Autodesk Inventor part; units mm, degrees
ref_plane "YZ Plane" through (0, 0, 0) normal (1, 0, 0) x (0, 1, 0)
ref_plane "XZ Plane" through (0, 0, 0) normal (0, 1, 0) x (-1, 0, 0)
ref_plane "XY Plane" through (0, 0, 0) normal (0, 0, 1) x (1, 0, 0)
sketch "Sketch5" plane through (0, 0, 0) normal (0, 1, 0) x (-1, 0, 0)
  line L0 (0, 0) -> (40, 0)
  line L1 (40, 0) -> (40, 150)
  line L2 (40, 150) -> (0, 150)
  line L3 (0, 150) -> (0, 0)
  line L4 (40, 150) -> (40, 140)
  line L5 (40, 140) -> (30, 140)
  circle A0 centre (30, 140) radius 2.75
  circle A1 centre (30, 10) radius 2.75
  circle A2 centre (10, 140) radius 2.75
  circle A3 centre (10, 10) radius 2.75
  line L6 (32.75, 140) -> (32.75, 10)
  line L7 (27.25, 10) -> (27.25, 140)
  line L8 (12.75, 140) -> (12.75, 10)
  line L9 (7.25, 10) -> (7.25, 140)
  dimension "d107" = 40
  dimension "d108" = 150
  dimension "d109" = 10
  dimension "d110" = 10
  dimension "d111" = 5.5
  dimension "d114" = 130
  dimension "d117" = 20
extrude "Extrusion3" add sketch "Sketch5" along normal blind 10
sketch "Sketch6" plane through (0, 10, 0) normal (0, 1, 0) x (1, 0, 0)
  arc A0 (-32.75, -140) -> (-27.25, -140) centre (-30, -140) ccw
  circle A1 centre (-30, -140) radius 4.5
  arc A2 (-27.25, -10) -> (-32.75, -10) centre (-30, -10) ccw
  circle A3 centre (-30, -10) radius 4.5
  arc A4 (-7.25, -10) -> (-12.75, -10) centre (-10, -10) ccw
  circle A5 centre (-10, -10) radius 4.5
  circle A6 centre (-10, -140) radius 4.5
  line L0 (-34.5, -140) -> (-34.5, -10)
  line L1 (-25.5, -10) -> (-25.5, -140)
  line L2 (-14.5, -140) -> (-14.5, -10)
  line L3 (-5.5, -10) -> (-5.5, -140)
  point P0 (0, 0)
  dimension "d122" = 9
  dimension "d123" = 9
  dimension "d124" = 9
  dimension "d125" = 9
extrude "Extrusion4" cut sketch "Sketch6" against normal blind 6
fillet "Fillet2" radius 5 4 edges at (0, 5, 150) (-40, 5, 150) (0, 5, 0) (-40, 5, 0)
properties part number "GARFO" material "Aluminium AW-7020"
Can you work these out from the model? Positions are in its coordinate system, mm. A direction names the side the tool comes from. Coordinates: 2 decimals unless noted, no trailing zeros. Write each loop counter-clockwise with the first axis right and the second up, starting at its lowest first coordinate (ties: lowest second). Pieces come first, ordered by that corner, then holes. Notation, with made-up numbers: (75.5, 37) - (81.5, 37) arc R11 ccw to (81.5, 44) - close; hole circle Ø10 at (24.5, -19). An arc over 180 degrees is marked (long way). Return JSON: item names as keys, results as strings.
Q1. If we section it at B-B (y = 5.25): Please give me the cut outline in (x, z), then the cut area to 3 significant figures.
Computed values:
{"outline": "(-40, 5) arc R5 ccw to (-35, 0) - (-5, 0) arc R5 ccw to (0, 5) - (0, 145) arc R5 ccw to (-5, 150) - (-35, 150) arc R5 ccw to (-40, 145) - close; hole (-34.5, 10) arc R4.5 ccw to (-25.5, 10) - (-25.5, 140) arc R4.5 ccw to (-34.5, 140) - close; hole (-14.5, 10) arc R4.5 ccw to (-5.5, 10) - (-5.5, 140) arc R4.5 ccw to (-14.5, 140) - close", "area": "3,510 mm2"}
Q2. Thinking about a two-plate mould opening in Z: for faces 1 (the cylindrical face through (-2, 5, 149)), 2 (the cylindrical face through (-1, 5, 2)), 3 (the flat face through (-33, 4, 74)), which applies, +Z half, -Z half, draft (parallel to the pull), parting line (faces both ways), or undercut?
Computed values:
{"face 1": "+Z half", "face 2": "-Z half", "face 3": "undercut"}
Q3. On a 3-axis mill with a long thin cutter (end or side, diameter ignored), from which of +Z, -Z, +X, -X, +Y, -Y can I reach the whole of each face in a straight line? I mean faces 4 (the flat face through (-20, 5, 150)), 5 (the cylindrical face through (-29.9, 7, 5.5)), 6 (the cylindrical face through (-9.94, 1.97, 142.75)). Say none if no direction works.
Computed values:
{"face 4": "+Z, +X, -X, +Y, -Y", "face 5": "+Y", "face 6": "+Y, -Y"}
Q4. If we section it at A-A (z = 104): Please give me the cut outline in (x, y).
Computed values:
{"outline": "(-40, 0) - (-32.75, 0) - (-32.75, 4) - (-34.5, 4) - (-34.5, 10) - (-40, 10) - close; (-27.25, 0) - (-12.75, 0) - (-12.75, 4) - (-14.5, 4) - (-14.5, 10) - (-25.5, 10) - (-25.5, 4) - (-27.25, 4) - close; (-7.25, 0) - (0, 0) - (0, 10) - (-5.5, 10) - (-5.5, 4) - (-7.25, 4) - close"}
Q5. I'm going to push a flat-ended pin straight in: pin 1 Ø4 at (x, z) = (-8.5, 115.5) entering from +Y. Where does the tip first touch, or does it pass through?
Computed values:
{"pin 1": "stops at y = 4"}
Q6. If we section it at C-C (x = -30): Please give me the cut outline in (y, z), then the cut area to 3 significant figures.
Computed values:
{"outline": "(0, 0) - (10, 0) - (10, 5.5) - (4, 5.5) - (4, 7.25) - (0, 7.25) - close; (0, 142.75) - (4, 142.75) - (4, 144.5) - (10, 144.5) - (10, 150) - (0, 150) - close", "area": "124 mm2"}
Q7. Please list where these lines run through material, in increasing order: L1, parallel to X at y = 8.5, z = 97; L2, parallel to X at y = 1.75, z = 25.5; L3, parallel to Y at x = -34, z = 13. Write a range as from..to.
Computed values:
{"L1": "x = -40..-34.5, -25.5..-14.5, -5.5..0", "L2": "x = -40..-32.75, -27.25..-12.75, -7.25..0", "L3": "y = 0..4"}
